The listing builds one solid part. Answer for the finished solid, in the listing's coordinates (mm). Face numbers are marked on the shaded views. A direction names the side the tool comes from. Give positions to 0.01 mm unless a question says otherwise; leave off trailing zeros. Write each loop counter-clockwise with the first axis right and the second up, starting at its lowest first coordinate (ties: lowest second). Pieces come first, ordered by that corner, then holes. Notation, with made-up numbers: (-35, 39) -> (8, 39) arc R23 ccw to (8, 76) -> close; hole circle Ø5 at (-11, 36). An arc over 180 degrees is marked (long way). Put each result on its own line as item: value. Start each with the question number.
1) For the marked faces 1 and 2, determine the directions among +Z, -Z, +X, -X, +Y, -Y from which every point of the face is accessible in a straight line to the end or side of a thin tool.
2) A cutting plane is placed at D-D (x = -20). Write down the section's boundary in (y, z).
3) A cutting plane is placed at B-B (x = 55). Write down the section's boundary in (y, z).
4) A cutting plane is placed at C-C (z = 14). Write down the section's boundary in (x, y), then the cut area to 3 significant figures.
5) A flat-ended cylindrical pin translates along its axis: pin 1 Ø8 at (x, y) = (7.5, -1.5) entering from +Z. Find the tip coordinate at first contact, or state that the pin passes through.
6) Find the intervals of material crossed by line 1 along Y through (x, z) = (56, 18.5); line 2 along X through (y, z) = (21.5, 7.25); line 3 along Z through (x, y) = (-5.5, -2), in increasing order. Write a range as from..to.
7) For a pull along X with two mould halves and no side action, classify the marked faces 3, 4 and 5 as released by +X, released by -X, zero draft, split by the parting line, or undercut.
8) A cutting plane is placed at A-A (y = -22.5). Write down the section's boundary in (x, z).
from build123d import *

# Parameters (mm, degrees)
F0_W     = 127
F0_H     = 88.9
F1_DEPTH = 25.4
F2_T     = -2.54
F3_R     = 8.89
F4_DEPTH = 1270
F5_R     = 2.54
F6_R     = 2.54


with BuildPart() as f1:
    # F0 (on Top) → F1 (new body)
    with BuildSketch(Plane.XY):
        with Locations((2.735384, 3.646639)):
            Rectangle(F0_W, F0_H)
    extrude(amount=F1_DEPTH)

    # F2
    f2_openings = [f1.faces().sort_by_distance(p)[0] for p in [
        (2.735384, 3.646639, 25.4),
    ]]
    offset(amount=F2_T, openings=f2_openings)

    # F3 (on face) → F4 (cut)
    with BuildSketch(Plane.XZ.offset(40.803361)):
        with Locations((-47.283076, 12.016155)):
            Circle(F3_R)
        with Locations((47.478464, 12.016155)):
            Circle(F3_R)
    extrude(amount=-F4_DEPTH, mode=Mode.SUBTRACT)

    # F5
    f5_edges = [f1.edges().sort_by_distance(p)[0] for p in [
        (66.235384, 3.646639, 0),
    ]]
    fillet(f5_edges, radius=F5_R)

    # F6
    f6_edges = [f1.edges().sort_by_distance(p)[0] for p in [
        (1.465384, -40.803361, 0),
        (66.235384, -40.803361, 13.97),
        (66.235384, 48.096639, 13.97),
        (1.465384, 48.096639, 0),
        (-60.764616, 3.646639, 0),
        (-60.764616, 48.096639, 12.7),
        (-60.764616, -40.803361, 12.7),
    ]]
    fillet(f6_edges, radius=F6_R)


solid = f1.part
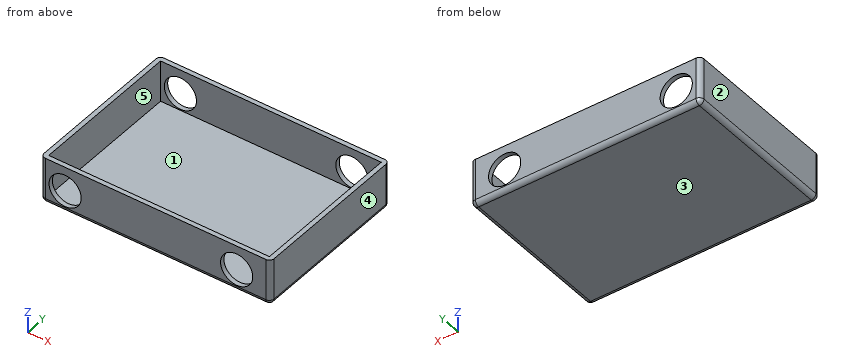
Reply:
1. face 1: +Z
1. face 2: +Z, -Z, -X, +Y, -Y
2. outline: (-40.8, 2.54) arc R2.54 ccw to (-38.26, 0) -> (45.56, 0) arc R2.54 ccw to (48.1, 2.54) -> (48.1, 25.4) -> (45.56, 25.4) -> (45.56, 2.54) -> (-38.26, 2.54) -> (-38.26, 25.4) -> (-40.8, 25.4) -> close
3. outline: (-40.8, 2.54) arc R2.54 ccw to (-38.26, 0) -> (45.56, 0) arc R2.54 ccw to (48.1, 2.54) -> (48.1, 7.28) -> (45.56, 7.28) -> (45.56, 2.54) -> (-38.26, 2.54) -> (-38.26, 7.28) -> (-40.8, 7.28) -> close; (-40.8, 16.76) -> (-38.26, 16.76) -> (-38.26, 25.4) -> (-40.8, 25.4) -> close; (45.56, 16.76) -> (48.1, 16.76) -> (48.1, 25.4) -> (45.56, 25.4) -> close
4. outline: (-60.76, -38.26) arc R2.54 ccw to (-58.22, -40.8) -> (-55.95, -40.8) -> (-55.95, -38.26) -> (-58.22, -38.26) -> (-58.22, 45.56) -> (-55.95, 45.56) -> (-55.95, 48.1) -> (-58.22, 48.1) arc R2.54 ccw to (-60.76, 45.56) -> close; (-38.62, -40.8) -> (38.81, -40.8) -> (38.81, -38.26) -> (-38.62, -38.26) -> close; (-38.62, 45.56) -> (38.81, 45.56) -> (38.81, 48.1) -> (-38.62, 48.1) -> close; (56.14, -40.8) -> (63.7, -40.8) arc R2.54 ccw to (66.24, -38.26) -> (66.24, 45.56) arc R2.54 ccw to (63.7, 48.1) -> (56.14, 48.1) -> (56.14, 45.56) -> (63.7, 45.56) -> (63.7, -38.26) -> (56.14, -38.26) -> close
4. area: 889 mm2
5. pin 1: stops at z = 2.54
6. line 1: y = -40.8..-38.26, 45.56..48.1
6. line 2: x = -60.76..-58.22, 63.7..66.24
6. line 3: z = 0..2.54
7. face 3: zero draft
7. face 4: released by +X
7. face 5: undercut
8. outline: (-60.76, 2.54) arc R2.54 ccw to (-58.22, 0) -> (63.7, 0) arc R2.54 ccw to (66.24, 2.54) -> (66.24, 25.4) -> (63.7, 25.4) -> (63.7, 2.54) -> (-58.22, 2.54) -> (-58.22, 25.4) -> (-60.76, 25.4) -> close
